from build123d import *

# Parameters (mm, degrees)
SKETCH_1_W      = 80
SKETCH_1_H      = 80
EXTRUDE_1_DEPTH = 4
FILLET_1_R      = 10


with BuildPart() as part:
    # Эскиз1 → Бобышка-Вытянуть1 (new body)
    with BuildSketch(Plane.XY):
        Rectangle(SKETCH_1_W, SKETCH_1_H)
        with BuildLine():
            Line((19, -20), (19, 20))
            ThreePointArc((19, 20), (25, 26), (31, 20))
            Line((31, 20), (31, -20))
            ThreePointArc((31, -20), (25, -26), (19, -20))
        make_face(mode=Mode.SUBTRACT)
        with BuildLine():
            Line((-31, -20), (-31, 20))
            ThreePointArc((-31, 20), (-25, 26), (-19, 20))
            Line((-19, 20), (-19, -20))
            ThreePointArc((-19, -20), (-25, -26), (-31, -20))
        make_face(mode=Mode.SUBTRACT)
    extrude(amount=EXTRUDE_1_DEPTH)

    # Скругление1
    fillet_1_edges = [part.edges().sort_by_distance(p)[0] for p in [
        (40, -40, 2),
        (-40, -40, 2),
        (-40, 40, 2),
        (40, 40, 2),
    ]]
    fillet(fillet_1_edges, radius=FILLET_1_R)


solid = part.part
Design review of the part built by this model. Coordinates are the model's own, in mm. A direction names the side the tool comes from. Coordinates: 2 decimals unless noted, no trailing zeros. Order: outer loops, then holes, each group sorted by start corner. A loop starts at its lowest first (then second) coordinate and runs counter-clockwise, first axis right, second up.
Item 1: For pin 1 Ø4 at (x, y) = (-21.5, 8) entering from +Z, flat-tipped, find the tip position at first contact; note if it passes through.
Item 2: For line 1 (X direction, y = -18.5, z = 1.9); line 2 (X direction, y = -21.5, z = 0.9); line 3 (Y direction, x = 27, z = 1.7), list the stretches that pass through material, from the lowest coordinate up.
Item 3: Take a section at B-B, the plane x = 25. Write out the cut boundary in (y, z), then the cut area to 3 significant figures.
Item 4: Take a section at A-A, the plane y = 18. Write out the cut boundary in (x, z).
Item 5: Take a section at C-C, the plane z = 1.3. Write out the cut boundary in (x, y).
Item 6: The part is to be moulded in two halves that separate along Y. For faces 3 (the flat face through (-31, 0, 2)), 4 (the cylindrical face through (25, 26, 2)), 5 (the cylindrical face through (-37.15, -36.99, 2.03)), 6 (the flat face through (-1, 1, 0)), say which applies: pulls with the +Y half, pulls with the -Y half, needs draft (parallel to the pull), parting line crosses it, or undercut.
Item 7: Take a section at D-D, the plane x = -34. Write out the cut boundary in (y, z).
Item 8: For faces 1 (the cylindrical face through (25, -26, 2)), 2 (the flat face through (40, 0, 2)), list the 3-axis set-ups (+Z, -Z, +X, -X, +Y, -Y) from which the entire face can be reached by the end or side of a thin tool; tool diameter is ignored.
The answers:
1. pin 1: passes through
2. line 1: x = -40 to -31, -19 to 19, 31 to 40
2. line 2: x = -40 to -30.81, -19.19 to 19.19, 30.81 to 40
2. line 3: y = -40 to -25.66, 25.66 to 40
3. outline: (-40, 0) - (-26, 0) - (-26, 4) - (-40, 4) - close; (26, 0) - (40, 0) - (40, 4) - (26, 4) - close
3. area: 112 mm2
4. outline: (-40, 0) - (-31, 0) - (-31, 4) - (-40, 4) - close; (-19, 0) - (19, 0) - (19, 4) - (-19, 4) - close; (31, 0) - (40, 0) - (40, 4) - (31, 4) - close
5. outline: (-40, -30) arc R10 ccw to (-30, -40) - (30, -40) arc R10 ccw to (40, -30) - (40, 30) arc R10 ccw to (30, 40) - (-30, 40) arc R10 ccw to (-40, 30) - close; hole (-31, -20) arc R6 ccw to (-19, -20) - (-19, 20) arc R6 ccw to (-31, 20) - close; hole (19, -20) arc R6 ccw to (31, -20) - (31, 20) arc R6 ccw to (19, 20) - close
6. face 3: undercut
6. face 4: undercut
6. face 5: pulls with the -Y half
6. face 6: needs draft
7. outline: (-39.17, 0) - (39.17, 0) - (39.17, 4) - (-39.17, 4) - close
8. face 1: +Z, -Z
8. face 2: +Z, -Z, +X, +Y, -Y
